```python
from build123d import *

# Parameters (mm, degrees)
SKETCH1_R                                        = 11.1
SKETCH1_R_2                                      = 1.5
BOSS_EXTRUDE1_DEPTH                              = 10
CBORE_FOR_M3_SHCS2_D                             = 3.4
CBORE_FOR_M3_SHCS2_CBORE_D                       = 6.5
CBORE_FOR_M3_SHCS2_CBORE_DEPTH                   = 3
BOSS_EXTRUDE2_DEPTH                              = 15
CBORE_FOR_M5_PAN_HEAD_MACHINE_SCREW1_D           = 5.5
CBORE_FOR_M5_PAN_HEAD_MACHINE_SCREW1_CBORE_D     = 11
CBORE_FOR_M5_PAN_HEAD_MACHINE_SCREW1_CBORE_DEPTH = 3.7


with BuildPart() as part:
    # Sketch1 → Boss-Extrude1 (new body)
    with BuildSketch(Plane(origin=(0, 0, 0), x_dir=(1, 0, 0), z_dir=(0, 1, 0))):
        with BuildLine():
            Line((-53.392463057, 46.326821798), (16.607536943, 46.326821798))
            ThreePointArc((16.607536943, 46.326821798), (23.678604755, 43.39788961), (26.607536943, 36.326821798))
            Line((26.607536943, 36.326821798), (26.607536943, -38.673178202))
            ThreePointArc((26.607536943, -38.673178202), (23.678604755, -45.744246014), (16.607536943, -48.673178202))
            Line((16.607536943, -48.673178202), (-53.392463057, -48.673178202))
            ThreePointArc((-53.392463057, -48.673178202), (-60.463530869, -45.744246014), (-63.392463057, -38.673178202))
            Line((-63.392463057, -38.673178202), (-63.392463057, 36.326821798))
            ThreePointArc((-63.392463057, 36.326821798), (-60.463530869, 43.39788961), (-53.392463057, 46.326821798))
        make_face()
        with Locations(Location((-18.392463057, -1.173178202, 0), (0, 0, 270))):
            Circle(SKETCH1_R, mode=Mode.SUBTRACT)
        with Locations(Location((-33.892463057, 14.326821798, 0), (0, 0, 270))):
            Circle(SKETCH1_R_2, mode=Mode.SUBTRACT)
        with Locations(Location((-2.892463057, 14.326821798, 0), (0, 0, 270))):
            Circle(SKETCH1_R_2, mode=Mode.SUBTRACT)
        with Locations(Location((-2.892463057, -16.673178202, 0), (0, 0, 270))):
            Circle(SKETCH1_R_2, mode=Mode.SUBTRACT)
        with Locations(Location((-33.892463057, -16.673178202, 0), (0, 0, 270))):
            Circle(SKETCH1_R_2, mode=Mode.SUBTRACT)
    extrude(amount=BOSS_EXTRUDE1_DEPTH)

    # CBORE for M3 SHCS2 (through all)
    with Locations(Plane(origin=(0, 0, 0), x_dir=(-1, 0, 0), z_dir=(0, -1, 0))):
        with Locations((33.892463057, 14.326821798), (33.892463057, -16.673178202), (2.892463057, -16.673178202), (2.892463057, 14.326821798)):
            CounterBoreHole(CBORE_FOR_M3_SHCS2_D / 2, CBORE_FOR_M3_SHCS2_CBORE_D / 2, CBORE_FOR_M3_SHCS2_CBORE_DEPTH)

    # Sketch14 → Boss-Extrude2 (add)
    with BuildSketch(Plane.XZ):
        with BuildLine():
            Line((-63.392463057, 21.173178202), (-63.392463057, 1.173178202))
            Line((-63.392463057, 1.173178202), (-45.24346378, 1.173178202))
            Line((-45.24346378, 1.173178202), (-45.24346378, 8.863568164))
            ThreePointArc((-45.24346378, 8.863568164), (-45.969681105, 12.604818608), (-48.042854757, 15.802676874))
            ThreePointArc((-48.042854757, 15.802676874), (-48.11206031, 15.853300063), (-48.194300833, 15.877561399))
            ThreePointArc((-48.194300833, 15.877561399), (-49.229807613, 16.702257146), (-48.943751594, 17.994762203))
            ThreePointArc((-48.943751594, 17.994762203), (-48.890905547, 18.264697041), (-49.118059331, 18.419805648))
            ThreePointArc((-49.118059331, 18.419805648), (-49.185476717, 18.420979486), (-49.252892133, 18.422261555))
            ThreePointArc((-49.252892133, 18.422261555), (-49.413697771, 18.367785226), (-49.502621898, 18.223152506))
            ThreePointArc((-49.502621898, 18.223152506), (-50.795128099, 17.229247149), (-51.970871232, 18.358870194))
            ThreePointArc((-51.970871232, 18.358870194), (-52.04340184, 18.512380567), (-52.197265304, 18.584159104))
            ThreePointArc((-52.197265304, 18.584159104), (-52.222766522, 18.586469356), (-52.248266326, 18.588795154))
            ThreePointArc((-52.248266326, 18.588795154), (-52.412550431, 18.545936584), (-52.511572027, 18.408020497))
            ThreePointArc((-52.511572027, 18.408020497), (-53.871728968, 17.508913587), (-54.963836872, 18.719583015))
            ThreePointArc((-54.963836872, 18.719583015), (-55.025224421, 18.877879234), (-55.173571608, 18.960457898))
            ThreePointArc((-55.173571608, 18.960457898), (-55.178476777, 18.961257271), (-55.183381852, 18.962057224))
            ThreePointArc((-55.183381852, 18.962057224), (-55.402367129, 18.890120336), (-55.46941862, 18.669590145))
            ThreePointArc((-55.46941862, 18.669590145), (-56.940189657, 17.214565757), (-57.748415424, 19.11904325))
            ThreePointArc((-57.748415424, 19.11904325), (-57.726719012, 19.348518158), (-57.901995791, 19.498209567))
            ThreePointArc((-57.901995791, 19.498209567), (-57.906837309, 19.499331791), (-57.911678694, 19.500454589))
            ThreePointArc((-57.911678694, 19.500454589), (-58.080270451, 19.480381142), (-58.197160956, 19.357244089))
            ThreePointArc((-58.197160956, 19.357244089), (-59.765354714, 18.68269589), (-60.54412767, 20.201827096))
            ThreePointArc((-60.54412767, 20.201827096), (-61.976998133, 20.661983137), (-63.392463057, 21.173178202))
        make_face()
        with BuildLine():
            Line((-63.392463057, 1.173178202), (-63.392463057, -18.826821798))
            ThreePointArc((-63.392463057, -18.826821798), (-61.976998133, -18.315626732), (-60.54412767, -17.855470691))
            ThreePointArc((-60.54412767, -17.855470691), (-59.765354714, -16.336339486), (-58.197160956, -17.010887685))
            ThreePointArc((-58.197160956, -17.010887685), (-58.080270451, -17.134024738), (-57.911678694, -17.154098184))
            ThreePointArc((-57.911678694, -17.154098184), (-57.906837309, -17.152975387), (-57.901995791, -17.151853162))
            ThreePointArc((-57.901995791, -17.151853162), (-57.726719012, -17.002161753), (-57.748415424, -16.772686846))
            ThreePointArc((-57.748415424, -16.772686846), (-56.940189657, -14.868209353), (-55.46941862, -16.323233741))
            ThreePointArc((-55.46941862, -16.323233741), (-55.402367129, -16.543763931), (-55.183381852, -16.615700819))
            ThreePointArc((-55.183381852, -16.615700819), (-55.178476777, -16.614900866), (-55.173571608, -16.614101494))
            ThreePointArc((-55.173571608, -16.614101494), (-55.025224421, -16.531522829), (-54.963836872, -16.373226611))
            ThreePointArc((-54.963836872, -16.373226611), (-53.871728968, -15.162557182), (-52.511572027, -16.061664092))
            ThreePointArc((-52.511572027, -16.061664092), (-52.412550431, -16.19958018), (-52.248266326, -16.242438749))
            ThreePointArc((-52.248266326, -16.242438749), (-52.222766522, -16.240112951), (-52.197265304, -16.2378027))
            ThreePointArc((-52.197265304, -16.2378027), (-52.04340184, -16.166024163), (-51.970871232, -16.012513789))
            ThreePointArc((-51.970871232, -16.012513789), (-50.795128099, -14.882890744), (-49.502621898, -15.876796101))
            ThreePointArc((-49.502621898, -15.876796101), (-49.413697771, -16.021428821), (-49.252892133, -16.07590515))
            ThreePointArc((-49.252892133, -16.07590515), (-49.185476717, -16.074623081), (-49.118059331, -16.073449243))
            ThreePointArc((-49.118059331, -16.073449243), (-48.890905547, -15.918340637), (-48.943751594, -15.648405799))
            ThreePointArc((-48.943751594, -15.648405799), (-49.229807613, -14.355900742), (-48.194300833, -13.531204995))
            ThreePointArc((-48.194300833, -13.531204995), (-48.11206031, -13.506943659), (-48.042854757, -13.45632047))
            ThreePointArc((-48.042854757, -13.45632047), (-45.969681105, -10.258462203), (-45.24346378, -6.517211759))
            Line((-45.24346378, -6.517211759), (-45.24346378, 1.173178202))
            Line((-45.24346378, 1.173178202), (-63.392463057, 1.173178202))
        make_face()
    extrude(amount=BOSS_EXTRUDE2_DEPTH)

    # CBORE for M5 Pan Head Machine Screw1 (through all)
    with Locations(Plane(origin=(0, 0, 0), x_dir=(-1, 0, 0), z_dir=(0, -1, 0))):
        with Locations((53.091066757, 35.326821798), (-11.607536943, 35.326821798), (-11.607536943, -37.673178202), (53.091066757, -37.673178202)):
            CounterBoreHole(CBORE_FOR_M5_PAN_HEAD_MACHINE_SCREW1_D / 2, CBORE_FOR_M5_PAN_HEAD_MACHINE_SCREW1_CBORE_D / 2, CBORE_FOR_M5_PAN_HEAD_MACHINE_SCREW1_CBORE_DEPTH)


solid = part.part
```
The listing builds one solid part. Answer for the finished solid, in the listing's coordinates (mm). A direction names the side the tool comes from. Round coordinates to 2 decimals unless told otherwise and drop trailing zeros. Write each loop counter-clockwise with the first axis right and the second up, starting at its lowest first coordinate (ties: lowest second). Pieces come first, ordered by that corner, then holes. Notation, with made-up numbers: (-27, -38) -> (8, -38) arc R24 cw to (8, -26) -> close; hole circle Ø7 at (25.25, -30). An arc over 180 degrees is marked (long way). Answer as a JSON object with one key per item and string values. Group by question number.
Q1. Each of these flat-tipped pins is pushed along its axis until it touches: pin 1 Ø5.5 at (x, z) = (10, -36) entering from -Y; pin 2 Ø10.5 at (x, z) = (-33.89, 16.67) entering from -Y; pin 3 Ø5 at (x, z) = (-33.89, -14.33) entering from -Y; pin 4 Ø2 at (x, z) = (-33.89, -14.33) entering from -Y. Where does it stop, or does it pass through?
Q2. Determine the mould class of faces 1 (the face through (23.756, 4.93, 45.666)), 2 (the face through (-63.392, 0, 2)), 3 (the face through (-4.3, 3, -12.9)), 4 (the face through (-55.63, 1.82, 42.55)) for opening direction X: pulls with the +X half, pulls with the -X half, needs draft (parallel to the pull), parting line crosses it, or undercut.
Q3. Section D-D (x = -44) is taken. Write down the section's boundary in (y, z).
Q4. Straight lines are drawn through the part: line 1 along Z through (x, y) = (12, 2.25); line 2 along Z through (x, y) = (9.5, 8); line 3 along Y through (x, z) = (-50.5, -33.5). For each, find the intervals that lie inside material, in ascending order.
Q5. Which of the six approach directions +Z, -Z, +X, -X, +Y, -Y give full straight-line access (tool end or side, diameter ignored) to faces 5 (the face through (-36.9, 1.5, 17.9)), 6 (the face through (-50.82, -7.395, -14.885)), 7 (the face through (-50.77, -7.4, 17.23)), 8 (the face through (-49.236, -7.395, -14.374))?
Q6. Section B-B (y = 7.75) is taken. Count the separate pieces of the cut face and the enclosed holes in it, plus the area to 3 significant figures.
Q7. Section A-A (z = -1) is taken. Write down the section's boundary in (x, y), plus the area to 3 significant figures.
Q8. Section C-C (z = 24) is taken. Write down the section's boundary in (x, y).
Check values:
{
 "1": {"pin 1": "y = 3.7", "pin 2": "y = 0", "pin 3": "y = 3", "pin 4": "through"},
 "2": {"face 1": "pulls with the +X half", "face 2": "pulls with the -X half", "face 3": "undercut", "face 4": "undercut"},
 "3": {"outline": "(0, -46.33) -> (10, -46.33) -> (10, 48.67) -> (0, 48.67) -> close"},
 "4": {"line 1": "-46.33 to -40.81, -29.84 to 32.19, 43.16 to 48.67", "line 2": "-46.33 to -37.09, -33.56 to 35.91, 39.44 to 48.67", "line 3": "3.7 to 10"},
 "5": {"face 5": "-Y", "face 6": "-Z, -Y", "face 7": "+Z, -Y", "face 8": "+X, -Y"},
 "6": {"separate pieces": "1", "enclosed holes": "9", "area": "7,950 mm^2"},
 "7": {"outline": "(-63.39, -15) -> (-45.24, -15) -> (-45.24, 0) -> (-29.28, 0) -> (-29.28, 10) -> (-63.39, 10) -> close; (-7.51, 0) -> (26.61, 0) -> (26.61, 10) -> (-7.51, 10) -> close", "area": "955 mm^2"},
 "8": {"outline": "(-63.39, 0) -> (26.61, 0) -> (26.61, 10) -> (-63.39, 10) -> close"}
}
